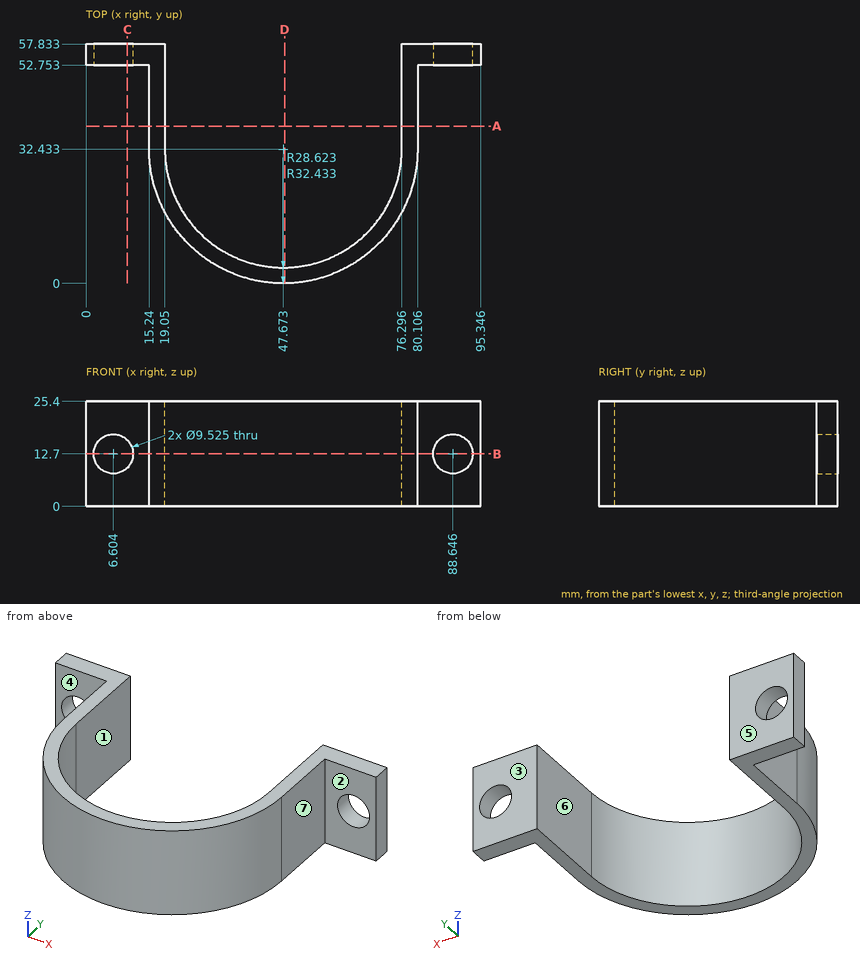
Geometry check sheet. Reference: drawing and pictorial views, mm from the part's lowest x, y, z. A direction names the side the tool comes from. Coordinates: 2 decimals unless noted, no trailing zeros. Order: outer loops, then holes, each group sorted by start corner. A loop starts at its lowest first (then second) coordinate and runs counter-clockwise, first axis right, second up. Notation, with made-up numbers: (-15.75, -17) - (7.25, -17) arc R18 cw to (7.25, 14) - close; hole circle Ø1 at (-38, -21.5). An arc over 180 degrees is marked (long way). Answer in a Markdown table with one row per item. Add a question column.
1) Gauge pin test, flat ends, axial feed: P1, Ø6, axis at y = 38, z = 12, coming from the +X side; P2, Ø12, axis at x = 88.5, z = 8.5, coming from the -Y side; P3, Ø5, axis at y = 29, z = 3, coming from the -X side. Record the tip position at first contact, or that the pin passes through.
2) Material ranges on line 1 along X through (y, z) = (51, 23); line 2 along Y through (x, z) = (48, 5); line 3 along Y through (x, z) = (5, 3), recorded low to high. Write a range as [from, to].
3) Set-up check for the marked faces 1, 2, 3 and 4: record each of +Z, -Z, +X, -X, +Y, -Y from which the full face is reachable in a straight line by a thin tool's end or side.
4) Cross-section at D-D, the plane x = 48. Record the cut outline in (y, z).
5) Cross-section at B-B, the plane z = 12.7. Record the cut outline in (x, y), then the cut area to 3 significant figures.
6) Cross-section at A-A, the plane y = 38. Record the cut outline in (x, z).
7) Cross-section at C-C, the plane x = 10. Record the cut outline in (y, z).
8) Release check for a two-part mould opening along X. For the marked faces 5, 6 and 7 record: +X half, -X half, draft (parallel to the pull), parting line (faces both ways), or undercut.
Check result:
| question | item | result |
|---|---|---|
| 1 | P1 | stops at x = 80.11 |
| 1 | P2 | stops at y = 52.75 |
| 1 | P3 | stops at x = 15.25 |
| 2 | line 1 | x = [15.24, 19.05], [76.3, 80.11] |
| 2 | line 2 | y = [0, 3.81] |
| 2 | line 3 | y = [52.75, 57.83] |
| 3 | face 1 | +Z, -Z, +Y |
| 3 | face 2 | +Z, -Z, +X, -Y |
| 3 | face 3 | +Z, -Z, +X, -X, +Y |
| 3 | face 4 | +Z, -Z, -X, -Y |
| 4 | outline | (0, 0) - (3.81, 0) - (3.81, 25.4) - (0, 25.4) - close |
| 5 | outline | (0, 52.75) - (1.84, 52.75) - (1.84, 57.83) - (0, 57.83) - close; (11.37, 52.75) - (15.24, 52.75) - (15.24, 32.43) arc R32.43 ccw to (80.11, 32.43) - (80.11, 52.75) - (83.88, 52.75) - (83.88, 57.83) - (76.3, 57.83) - (76.3, 32.43) arc R28.62 cw to (19.05, 32.43) - (19.05, 57.83) - (11.37, 57.83) - close; (93.41, 52.75) - (95.35, 52.75) - (95.35, 57.83) - (93.41, 57.83) - close |
| 5 | area | 617 mm² |
| 6 | outline | (15.24, 0) - (19.05, 0) - (19.05, 25.4) - (15.24, 25.4) - close; (76.3, 0) - (80.11, 0) - (80.11, 25.4) - (76.3, 25.4) - close |
| 7 | outline | (52.75, 0) - (57.83, 0) - (57.83, 9.36) - (52.75, 9.36) - close; (52.75, 16.04) - (57.83, 16.04) - (57.83, 25.4) - (52.75, 25.4) - close |
| 8 | face 5 | draft |
| 8 | face 6 | undercut |
| 8 | face 7 | +X half |
